Verification items for the finished model (mm, model axes). Face numbers are marked on the shaded views. A direction names the side the tool comes from. Give positions to 0.01 mm unless a question says otherwise; leave off trailing zeros. Order: outer loops, then holes, each group sorted by start corner. A loop starts at its lowest first (then second) coordinate and runs counter-clockwise, first axis right, second up. Notation, with made-up numbers: (29, 83) -> (71, 83) arc R14 ccw to (71, 104) -> close; hole circle Ø1 at (34.5, 35). An arc over 180 degrees is marked (long way). Write each question's results on one line, items separated by ' | '. Start each with the question number.
1. Set-up check for the marked faces 1, 2 and 3: record each of +Z, -Z, +X, -X, +Y, -Y from which the full face is reachable in a straight line by a thin tool's end or side.
2. Mould release check, pull along X, two halves, no side actions. Record for the marked faces 4, 5 and 6: +X half, -X half, draft (parallel to the pull), parting line (faces both ways), or undercut.
3. Cross-section at B-B, the plane x = 7. Enter the section's corners in (y, z).
4. Material ranges on L1, parallel to X at y = 8.5, z = 20; L2, parallel to X at y = -7, z = 15, recorded low to high. Write a range as from..to.
5. Cross-section at A-A, the plane x = 0. Enter the section's corners in (y, z), then the cut area to 3 significant figures.
6. Depth check by flat-ended pin: pin 1 Ø3 at (x, z) = (1, 14.5) entering from -Y; pin 2 Ø1.7 at (y, z) = (-1, 23.5) entering from +X; pin 3 Ø1 at (y, z) = (-2.5, 24) entering from +X. Enter the tip coordinate at first touch or a pass-through.
from build123d import *

# Parameters (mm, degrees)
BOSS_EXTRUDE1_DEPTH = 45.32
SKETCH2_R           = 2.1
CUT_EXTRUDE1_DEPTH  = 46.32
SKETCH3_R           = 2.1
CUT_EXTRUDE2_DEPTH  = 14.900660172


with BuildPart() as part:
    # Sketch1 → Boss-Extrude1 (new body)
    with BuildSketch(Plane.XY):
        Polygon((-3.1, 10), (-3.1, 8.200660172), (-5.5, 8.200660172), (-5.5, 6.560660172), (-2.84, 3.900660172), (2.84, 3.900660172), (5.5, 6.560660172), (5.5, 8.200660172), (3.1, 8.200660172), (3.1, 10), (10, 10), (10, 3.1), (8.200660172, 3.1), (8.200660172, 5.5), (6.560660172, 5.5), (3.900660172, 2.84), (3.900660172, -2.84), (6.560660172, -5.5), (8.200660172, -5.5), (8.200660172, -3.1), (10, -3.1), (10, -10), (3.1, -10), (3.1, -8.200660172), (5.5, -8.200660172), (5.5, -6.560660172), (2.84, -3.900660172), (-2.84, -3.900660172), (-5.5, -6.560660172), (-5.5, -8.200660172), (-3.1, -8.200660172), (-3.1, -10), (-10, -10), (-10, -3.1), (-8.200660172, -3.1), (-8.200660172, -5.5), (-6.560660172, -5.5), (-3.900660172, -2.84), (-3.900660172, 2.84), (-6.560660172, 5.5), (-8.200660172, 5.5), (-8.200660172, 3.1), (-10, 3.1), (-10, 10), align=None)
    extrude(amount=BOSS_EXTRUDE1_DEPTH)

    # Sketch2 → Cut-Extrude1 (cut, through all)
    with BuildSketch(Plane.XY.offset(45.32)):
        Circle(SKETCH2_R)
    extrude(amount=-CUT_EXTRUDE1_DEPTH, mode=Mode.SUBTRACT)

    # Sketch3 → Cut-Extrude2 (cut, through all)
    with BuildSketch(Plane(origin=(0, 3.900660172, 0), x_dir=(1, 0, 0), z_dir=(0, 1, 0))):
        with Locations((0, -22.66)):
            Circle(SKETCH3_R)
    extrude(amount=-CUT_EXTRUDE2_DEPTH, mode=Mode.SUBTRACT)


solid = part.part
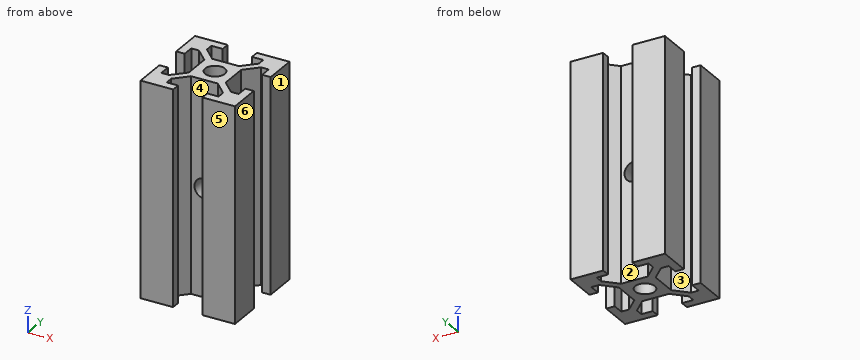
Results below:
1) face 1: +Z, -Z, +X, +Y, -Y | face 2: +Z, -Z, +Y | face 3: +Z, -Z
2) face 4: undercut | face 5: draft | face 6: +X half
3) outline: (-10, 0) -> (-5.5, 0) -> (-5.5, 45.32) -> (-10, 45.32) -> close; (5.5, 0) -> (10, 0) -> (10, 45.32) -> (5.5, 45.32) -> close
4) L1: x = -10..-3.1, 3.1..10 | L2: x = -10..-5.5, 5.5..10
5) outline: (-3.9, 0) -> (-2.1, 0) -> (-2.1, 20.56) -> (-3.9, 20.56) -> close; (-3.9, 24.76) -> (-2.1, 24.76) -> (-2.1, 45.32) -> (-3.9, 45.32) -> close; (2.1, 0) -> (3.9, 0) -> (3.9, 20.56) -> (2.1, 20.56) -> close; (2.1, 24.76) -> (3.9, 24.76) -> (3.9, 45.32) -> (2.1, 45.32) -> close | area: 148 mm²
6) pin 1: stops at y = -3.9 | pin 2: stops at x = 3.9 | pin 3: stops at x = 4.06
